Answer from the drawing. Dimensions are ordinates in mm from the lowest x, y and z of the part. A direction names the side the tool comes from. Coordinates: 2 decimals unless noted, no trailing zeros. Loops run counter-clockwise (first coordinate to the right, second up) from the corner with the lowest first, then second, coordinate; pieces in that order, holes last. Notation, with made-up numbers: (-15, 78.25) -> (20, 78.25) arc R14 ccw to (20, 91.25) -> close; hole circle Ø8 at (-12.75, 88.25). An arc over 180 degrees is marked (long way). Use a Markdown table: item, result.
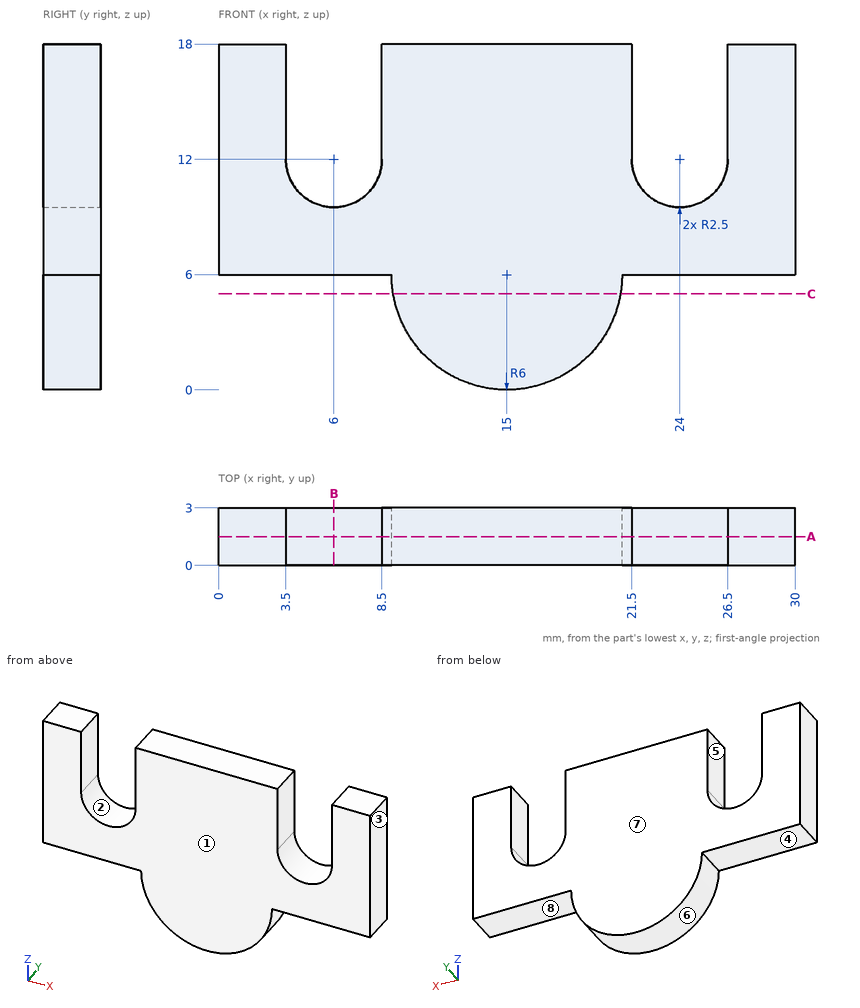
Q1. Section A-A on y = 1.5 is taken. Determine the outline of the cut face in (x, z), and give its area (3 significant figures).
Solved:
| item | result |
|---|---|
| outline | (0, 6) -> (9, 6) arc R6 ccw to (21, 6) -> (30, 6) -> (30, 18) -> (26.5, 18) -> (26.5, 12) arc R2.5 cw to (21.5, 12) -> (21.5, 18) -> (8.5, 18) -> (8.5, 12) arc R2.5 cw to (3.5, 12) -> (3.5, 18) -> (0, 18) -> close |
| area | 337 mm² |
Q2. Consider line 1 (X direction, y = 1.1, z = 16.25); line 2 (Z direction, x = 8.75, y = 0.7); line 3 (X direction, y = 2.05, z = 1). Determine where each line is inside the solid, lowest interval first. Write a range as [from, to].
Solved:
| item | result |
|---|---|
| line 1 | [0, 3.5], [8.5, 21.5], [26.5, 30] |
| line 2 | [6, 18] |
| line 3 | [11.68, 18.32] |
Q3. Section B-B on x = 6 is taken. Determine the outline of the cut face in (y, z), and give its area (3 significant figures).
Solved:
| item | result |
|---|---|
| outline | (0, 6) -> (3, 6) -> (3, 9.5) -> (0, 9.5) -> close |
| area | 10.5 mm² |
Q4. Determine the mould class of the marked faces 1, 2 and 3 for opening direction X: pulls with the +X half, pulls with the -X half, needs draft (parallel to the pull), parting line crosses it, or undercut.
Solved:
| item | result |
|---|---|
| face 1 | needs draft |
| face 2 | undercut |
| face 3 | pulls with the +X half |
Q5. Given pin 1 Ø1.5 at (x, y) = (25.5, 1) entering from -Z; pin 2 Ø1.5 at (y, z) = (1, 14) entering from -X, each flat-ended and moving along its own axis, determine where each tip first touches the part or whether it passes through.
Solved:
| item | result |
|---|---|
| pin 1 | z = 6 |
| pin 2 | x = 0 |
Q6. For the marked faces 4, 5, 6, 7 and 8, determine the directions among +Z, -Z, +X, -X, +Y, -Y from which every point of the face is accessible in a straight line to the end or side of a thin tool.
Solved:
| item | result |
|---|---|
| face 4 | -Z, -X, +Y, -Y |
| face 5 | +Z, +Y, -Y |
| face 6 | -Z, +Y, -Y |
| face 7 | +Z, -Z, +X, -X, +Y |
| face 8 | -Z, +X, +Y, -Y |
Q7. Section C-C on z = 5 is taken. Determine the outline of the cut face in (x, y), and give its area (3 significant figures).
Solved:
| item | result |
|---|---|
| outline | (9.08, 0) -> (20.92, 0) -> (20.92, 3) -> (9.08, 3) -> close |
| area | 35.5 mm² |
